```python
from build123d import *

# Parameters (mm, degrees)
SKETCH_1_W          = 15
SKETCH_1_H          = 15
SKETCH_1_W_2        = 13
SKETCH_1_H_2        = 13
EXTRUDE_1_DEPTH     = 185
SKETCH_2_R          = 1.45
CUT_EXTRUDE_1_DEPTH = 186.758579883
SKETCH_3_R          = 1.45
CUT_EXTRUDE_2_DEPTH = 186.758579883


with BuildPart() as part:
    # 草图1 → 凸台-拉伸1 (new body)
    with BuildSketch(Plane(origin=(0, 0, 0), x_dir=(0, 0, -1), z_dir=(1, 0, 0))):
        Rectangle(SKETCH_1_W, SKETCH_1_H)
        Rectangle(SKETCH_1_W_2, SKETCH_1_H_2, mode=Mode.SUBTRACT)
    extrude(amount=EXTRUDE_1_DEPTH)

    # 草图2 → 切除-拉伸1 (cut, through all)
    with BuildSketch(Plane.XZ.offset(7.5)):
        with Locations(Location((181, 0, 0), (0, 0, 270))):
            Circle(SKETCH_2_R)
        with Locations(Location((171, 0, 0), (0, 0, 270))):
            Circle(SKETCH_2_R)
        with Locations(Location((127.5, 0, 0), (0, 0, 270))):
            Circle(SKETCH_2_R)
        with Locations(Location((100, 0, 0), (0, 0, 270))):
            Circle(SKETCH_2_R)
        with Locations(Location((75, 0, 0), (0, 0, 270))):
            Circle(SKETCH_2_R)
        with Locations(Location((19, 0, 0), (0, 0, 270))):
            Circle(SKETCH_2_R)
        with Locations(Location((9, 0, 0), (0, 0, 270))):
            Circle(SKETCH_2_R)
        with Locations(Location((143, 0, 0), (0, 0, 270))):
            Circle(SKETCH_2_R)
        with Locations(Location((38.322949017, 0, 0), (0, 0, 270))):
            Circle(SKETCH_2_R)
        with Locations(Location((53.322949017, 0, 0), (0, 0, 270))):
            Circle(SKETCH_2_R)
    extrude(amount=-CUT_EXTRUDE_1_DEPTH, mode=Mode.SUBTRACT)

    # 草图3 → 切除-拉伸2 (cut, through all)
    with BuildSketch(Plane.XY.offset(7.5)):
        with Locations((14, 0)):
            Circle(SKETCH_3_R)
    extrude(amount=-CUT_EXTRUDE_2_DEPTH, mode=Mode.SUBTRACT)


solid = part.part
```
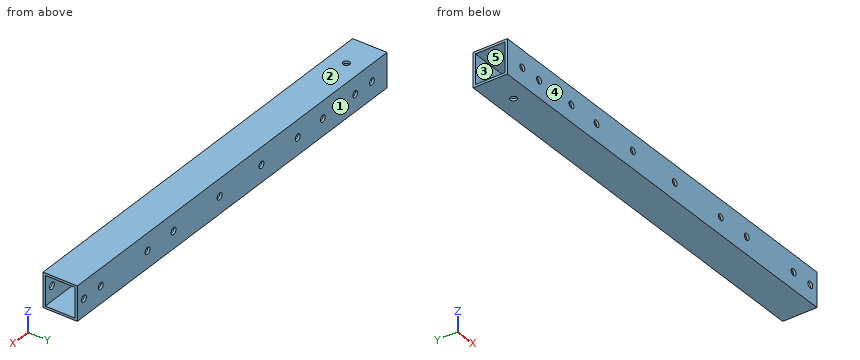
Part model, mm, in its own coordinate system. Face numbers are marked on the shaded views. A direction names the side the tool comes from. Give positions to 0.01 mm unless a question says otherwise; leave off trailing zeros. Write each loop counter-clockwise with the first axis right and the second up, starting at its lowest first coordinate (ties: lowest second). Pieces come first, ordered by that corner, then holes. Notation, with made-up numbers: (51, 79) -> (59, 79) arc R18 ccw to (59, 112) -> close; hole circle Ø4 at (-11, 45.5). An arc over 180 degrees is marked (long way). Put each result on its own line as item: value. Start each with the question number.
Item 1: Pin check, flat tips, straight feed: pin 1 Ø3.5 at (x, z) = (143, 0) entering from +Y; pin 2 Ø2.5 at (x, z) = (75, 0) entering from +Y. Stop position of each tip, or through.
Item 2: Cut at A-A (y = 3). List the corners of the cut face in (x, z).
Item 3: Which spindle directions (+Z, -Z, +X, -X, +Y, -Y) get a long thin tool onto all of the face, cutting with end or side? Do the marked faces 4 and 5. Say none if no direction does.
Item 4: Wall check: L1, parallel to Z at x = 143, y = 7; L2, parallel to Z at x = 121.5, y = 0.75. Give the ranges that are in metal, low to high. Write a range as [from, to].
Item 5: Pull direction Z, two halves, no side cores. Call the marked faces 1, 2 and 3: pulls with the +Z half, pulls with the -Z half, needs draft (parallel to the pull), parting line crosses it, or undercut.
Answer list:
1. pin 1: stops at y = 7.5
1. pin 2: passes through
2. outline: (0, -7.5) -> (185, -7.5) -> (185, -6.5) -> (0, -6.5) -> close; (0, 6.5) -> (185, 6.5) -> (185, 7.5) -> (0, 7.5) -> close
3. face 4: +Z, -Z, +X, -X, -Y
3. face 5: +X, -X
4. L1: z = [-7.5, -1.45], [1.45, 7.5]
4. L2: z = [-7.5, -6.5], [6.5, 7.5]
5. face 1: needs draft
5. face 2: pulls with the +Z half
5. face 3: undercut
